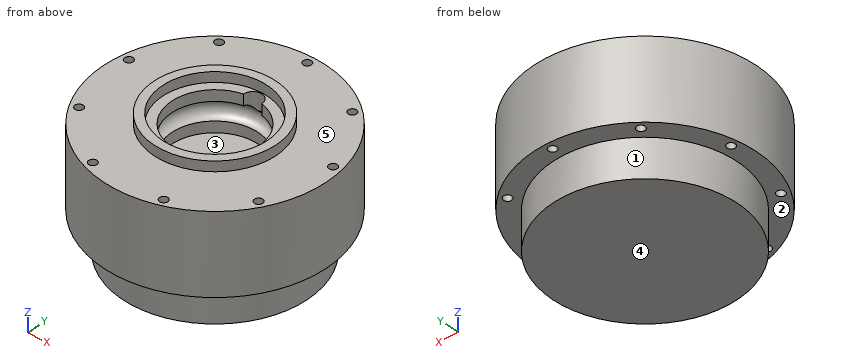
```python
from build123d import *

# Parameters (mm, degrees)
F_3_0MM_DOWEL_HOLE3_D   = 2.9
CUT_EXTRUDE1_DEPTH      = 70.306384987
CUT_EXTRUDE1_DEPTH_BACK = 6
SKETCH15_R              = 3.2


with BuildPart() as part:
    # Sketch12 → Revolve2 (revolve)
    with BuildSketch(Plane(origin=(0, 0, 0), x_dir=(0, 0, -1), z_dir=(1, 0, 0)), mode=Mode.PRIVATE) as revolve2_sk:
        with BuildLine():
            ThreePointArc((-17.809780572, 15.25), (-21, 18.2), (-24.190219428, 15.25))
            Line((-24.190219428, 15.25), (-28, 15.25))
            Line((-28, 15.25), (-28, 18.5))
            Line((-28, 18.5), (-31.5, 18.5))
            Line((-31.5, 18.5), (-31.5, 21.5))
            Line((-31.5, 21.5), (-28, 21.5))
            Line((-28, 21.5), (-28, 39.25))
            Line((-28, 39.25), (0, 39.25))
            Line((0, 39.25), (0, 32.5))
            Line((0, 32.5), (13.5, 32.5))
            Line((13.5, 32.5), (13.5, 0))
            Line((13.5, 0), (-14, 0))
            Line((-14, 0), (-14, 15.25))
            Line((-14, 15.25), (-17.809780572, 15.25))
        make_face()
    revolve(revolve2_sk.sketch.rotate(Axis((0, 0, 41.148719721), (0, 0, -1)), 90), axis=Axis((0, 0, 41.148719721), (0, 0, -1)))

    # Ø3.0mm Dowel Hole3 (through all)
    with Locations(Plane.XY.offset(28)):
        with Locations((-23.461747754, 27.960622174), (0, 36.5), (23.461747754, 27.960622174), (35.945482985, 6.338158485), (31.609927238, -18.25), (12.483735231, -34.298780659), (-12.483735231, -34.298780659), (-31.609927238, -18.25), (-35.945482985, 6.338158485)):
            Hole(F_3_0MM_DOWEL_HOLE3_D / 2)

    # Sketch15 → Cut-Extrude1 (cut, two sides: drawn at the far end of the back side and taken through both)
    with BuildSketch(Plane.XY.offset(28).offset(-CUT_EXTRUDE1_DEPTH_BACK)):
        with Locations((0, 15)):
            Circle(SKETCH15_R)
    extrude(amount=CUT_EXTRUDE1_DEPTH + CUT_EXTRUDE1_DEPTH_BACK, mode=Mode.SUBTRACT)


solid = part.part
```
Can you work these out from the model? Positions are in its coordinate system, mm. Face numbers are marked on the shaded views. A direction names the side the tool comes from. Round coordinates to 2 decimals unless told otherwise and drop trailing zeros. Loops run counter-clockwise (first coordinate to the right, second up) from the corner with the lowest first, then second, coordinate; pieces in that order, holes last. Notation, with made-up numbers: M 30.5,13.5 L 83.5,13.5 A36 ccw 83.5,47.5 Z; hole C -29,47.5 d8. An arc over 180 degrees is marked long. Answer as a JSON object with one key per item and string values. Group by question number.
Q1. Imagine slicing it at C-C, the plane y = 36.5. Please give me the cut outline in (x, z).
Q2. Will these pins go through, and if not, where does the flat tip stop? pin 1 (12 mm diameter, centred on x = 14, z = 15.5, fed in from +Y); pin 2 (2 mm diameter, centred on x = -1, y = -5.5, fed in from +Z); pin 3 (12 mm diameter, centred on x = -29, y = -30.5, fed in from -Z); pin 4 (2.5 mm diameter, centred on x = -23.46, y = 27.96, fed in from +Z).
Q3. We'd pull the mould along X, two halves only. Please class the marked faces 1, 2 and 3: +X half, -X half, draft (parallel to the pull), parting line (faces both ways), or undercut.
Q4. Please list where these lines run through material, in increasing order: L1, parallel to X at y = -34.5, z = 21; L2, parallel to Z at x = 24, y = -25.5; L3, parallel to Z at x = 17.5, y = -18.5.
Q5. On a 3-axis mill with a long thin cutter (end or side, diameter ignored), from which of +Z, -Z, +X, -X, +Y, -Y can I reach the whole of each face in a straight line? I mean the marked faces 4 and 5. Say none if no direction works.
Q6. Imagine slicing it at B-B, the plane z = 27. Count the separate pieces of the cut face and the enclosed holes in it, then the cut area to 3 significant figures.
Findings:
{
 "1": {"outline": "M -14.43,0 L -1.45,0 L -1.45,28 L -14.43,28 Z; M 1.45,0 L 14.43,0 L 14.43,28 L 1.45,28 Z"},
 "2": {"pin 1": "stops at y = 38.43", "pin 2": "stops at z = 14", "pin 3": "stops at z = 0", "pin 4": "passes through"},
 "3": {"face 1": "parting line", "face 2": "draft", "face 3": "undercut"},
 "4": {"L1": "x = -18.72 to -13.92, -11.05 to 11.05, 13.92 to 18.72", "L2": "z = 0 to 28", "L3": "z = -13.5 to 28"},
 "5": {"face 4": "-Z, +X, -X, +Y, -Y", "face 5": "+Z"},
 "6": {"separate pieces": "1", "enclosed holes": "10", "area": "4,030 mm2"}
}
